Model file for the job. Use its own axes, mm. A direction names the side the tool comes from. Coordinates: 2 decimals unless noted, no trailing zeros. Loops run counter-clockwise (first coordinate to the right, second up) from the corner with the lowest first, then second, coordinate; pieces in that order, holes last. Notation, with made-up numbers: M 10.5,-34 L 31.5,-34 A23 cw 31.5,-1 Z; hole C 72,40 d11. An arc over 180 degrees is marked long. One line per question, with ' | ' between items. Start each with the question number.
```python
from build123d import *

# Parameters (mm, degrees)
SKETCH1_R           = 4.318
BOSS_EXTRUDE1_DEPTH = 10.16
BOSS_EXTRUDE2_DEPTH = 15.24
SKETCH3_R           = 12.7
BOSS_EXTRUDE3_DEPTH = 25.4
EXTRUDE_THIN1_DEPTH = 2.54
SKETCH5_R           = 1.27
CUT_EXTRUDE1_DEPTH  = 0.254


with BuildPart() as part:
    # Sketch1 → Boss-Extrude1 (new body)
    with BuildSketch(Plane(origin=(0, 0, 0), x_dir=(1, 0, 0), z_dir=(0, 1, 0))):
        Circle(SKETCH1_R)
    extrude(amount=BOSS_EXTRUDE1_DEPTH)

    # Sketch2 → Boss-Extrude2 (add)
    with BuildSketch(Plane(origin=(0, 10.16, 0), x_dir=(1, 0, 0), z_dir=(0, 1, 0))):
        Polygon((0, 14.664696837), (-12.7, 7.332348419), (-12.7, -7.332348419), (0, -14.664696837), (12.7, -7.332348419), (12.7, 7.332348419), align=None)
    extrude(amount=BOSS_EXTRUDE2_DEPTH)

    # Sketch3 → Boss-Extrude3 (add)
    with BuildSketch(Plane(origin=(0, 25.4, 0), x_dir=(1, 0, 0), z_dir=(0, 1, 0))):
        Circle(SKETCH3_R)
    extrude(amount=BOSS_EXTRUDE3_DEPTH)

    # Sketch4 → Extrude-Thin1 (add, symmetric)
    with BuildSketch(Plane.XY):
        Polygon((7.62, 50.8), (7.62, 62.23), (11.43, 66.04), (11.609605122, 65.860394878), (7.874, 62.124789755), (7.874, 50.8), align=None)
    extrude_thin1 = extrude(amount=EXTRUDE_THIN1_DEPTH, both=True)

    # Sketch5 → Cut-Extrude1 (cut)
    with BuildSketch(Plane(origin=(-27.305, 27.305, 0), x_dir=(0, 0, 1), z_dir=(-0.707106781, 0.707106781, 0))):
        with Locations((0, 52.085485502)):
            Circle(SKETCH5_R)
    cut_extrude1 = extrude(amount=-CUT_EXTRUDE1_DEPTH, mode=Mode.SUBTRACT)

    # Mirror1: Extrude-Thin1, Cut-Extrude1 across plane
    add(extrude_thin1.mirror(Plane(origin=(0, 0, 0), x_dir=(0, 0, 1), z_dir=(1, 0, 0))))
    add(cut_extrude1.mirror(Plane(origin=(0, 0, 0), x_dir=(0, 0, 1), z_dir=(1, 0, 0))), mode=Mode.SUBTRACT)


solid = part.part
```
(1) Two-plate mould, pull along X, no slides. Class faces 1 (the face through (-11.4, 25.4, -6.3)), 2 (the face through (-2.75, 37.92, 12.4)), 3 (the face through (7.62, 56, 0)): pulls with the +X half, pulls with the -X half, needs draft (parallel to the pull), parting line crosses it, or undercut.
(2) 3-axis set-ups, long thin cutter, end or side, ignore diameter. For faces 4 (the face through (-7.62, 56, 0)), 5 (the face through (-10.6, 64.85, 1.16)), 6 (the face through (-3, 10.16, -3.5)), 7 (the face through (10.6, 64.85, 1.16)), 8 (the face through (0, 25.4, 13)): which of +Z, -Z, +X, -X, +Y, -Y reach the whole face in a straight line?
(3) Band-saw the part on A-A on y = 52.5. Write the cut outline in (x, z).
(4) Band-saw the part on D-D on x = 1.5. Write the cut outline in (y, z), then the cut area to 3 significant figures.
(5) Band-saw the part on B-B on y = 13. Write the cut outline in (x, z), then the cut area to 3 significant figures.
(6) Drill centre lines: line 1 (Y direction, x = 11.25, z = -7.75); line 2 (Z direction, x = -0.5, y = 47.5); line 3 (Y direction, x = -1.25, z = 2.75). Where is each one in solid material? Low to high. Write a range as [from, to].
(7) Pin check, flat tips, straight feed: P1, Ø5.5, axis at y = 56.5, z = 0, coming from the -X side; P2, Ø3, axis at x = -5.5, y = 41.5, coming from the -Z side; P3, Ø1.5, axis at y = 54.5, z = -1, coming from the +X side; P4, Ø2, axis at x = -10, y = 62, coming from the -Z side. Stop position of each tip, or through.
(8) Band-saw the part on C-C on z = -9.5. Write the cut outline in (x, y).
Computed values:
1) face 1: needs draft | face 2: parting line crosses it | face 3: undercut
2) face 4: +Z, -Z, +Y | face 5: +Z, -Z, -X | face 6: -Y | face 7: +Z, -Z, +X | face 8: +Z, +Y
3) outline: M -7.87,-2.54 L -7.62,-2.54 L -7.62,2.54 L -7.87,2.54 Z; M 7.62,-2.54 L 7.87,-2.54 L 7.87,2.54 L 7.62,2.54 Z
4) outline: M 0,-4.05 L 10.16,-4.05 L 10.16,-13.8 L 25.4,-13.8 L 25.4,-12.61 L 50.8,-12.61 L 50.8,12.61 L 25.4,12.61 L 25.4,13.8 L 10.16,13.8 L 10.16,4.05 L 0,4.05 Z | area: 1,140 mm^2
5) outline: M -12.7,-7.33 L 0,-14.66 L 12.7,-7.33 L 12.7,7.33 L 0,14.66 L -12.7,7.33 Z | area: 559 mm^2
6) line 1: [10.16, 25.4] | line 2: [-12.69, 12.69] | line 3: [0, 50.8]
7) P1: x = -7.87 | P2: z = -12.05 | P3: x = 7.87 | P4: through
8) outline: M -8.95,10.16 L 8.95,10.16 L 8.95,25.4 L 8.43,25.4 L 8.43,50.8 L -8.43,50.8 L -8.43,25.4 L -8.95,25.4 Z
